Verification items for the finished model (mm, model axes). Face numbers are marked on the shaded views. A direction names the side the tool comes from. Round coordinates to 2 decimals unless told otherwise and drop trailing zeros. Write each loop counter-clockwise with the first axis right and the second up, starting at its lowest first coordinate (ties: lowest second). Pieces come first, ordered by that corner, then holes. Notation, with made-up numbers: (60, 3) - (110, 3) arc R21 ccw to (110, 8) - close; hole circle Ø3 at (-39.5, -38.5). An arc over 180 degrees is marked (long way). Answer as a JSON object with one key per item and string values.
```python
from build123d import *

# Parameters (mm, degrees)
BOSS_EXTRUDE1_DEPTH = 35.56
SKETCH3_W           = 35.56
SKETCH3_H           = 6.35
BOSS_EXTRUDE2_DEPTH = 50.8
BOSS_EXTRUDE4_DEPTH = 35.56
CUT_EXTRUDE1_DEPTH  = 45.72
FILLET5_R           = 2.54


with BuildPart() as part:
    # Sketch2 → Boss-Extrude1 (new body)
    with BuildSketch(Plane.XY):
        Polygon((0, 0), (-114.3, 0), (-33.47769491, 80.82230509), (-28.98756685, 76.332177029), (-98.969743879, 6.35), (0, 6.35), align=None)
    extrude(amount=BOSS_EXTRUDE1_DEPTH)

    # Sketch3 → Boss-Extrude2 (add)
    with BuildSketch(Plane(origin=(-57.15, 57.15, 0), x_dir=(0, 0, 1), z_dir=(-0.707106781186544, 0.7071067811865511, 0))):
        with Locations((17.78, -42.08730509)):
            Rectangle(SKETCH3_W, SKETCH3_H)
    extrude(amount=BOSS_EXTRUDE2_DEPTH)

    # Sketch5 → Boss-Extrude4 (add)
    with BuildSketch(Plane.XY.offset(35.56)):
        Polygon((-98.969743879, 6.35), (-63.978655364, 41.341088515), (-63.978655364, 6.35), align=None)
    extrude(amount=-BOSS_EXTRUDE4_DEPTH)

    # Sketch6 → Cut-Extrude1 (cut)
    with BuildSketch(Plane(origin=(0, 0, 0), x_dir=(-1, 0, 0), z_dir=(0, 0, -1))):
        Polygon((67.153655364, 42.656216575), (67.153655364, 9.525), (100.284871939, 9.525), align=None)
    extrude(amount=-CUT_EXTRUDE1_DEPTH, mode=Mode.SUBTRACT)

    # Fillet5
    fillet5_edges = [part.edges().sort_by_distance(p)[0] for p in [
        (0, 0, 17.78),
        (-114.3, 0, 17.78),
        (-33.47769491, 80.82230509, 17.78),
        (-28.98756685, 76.332177029, 17.78),
        (0, 6.35, 17.78),
        (-31.23263088, 78.577241059, 35.56),
        (-101.727641431, 12.572358569, 0),
        (-101.727641431, 12.572358569, 35.56),
        (-59.071424855, 55.228575145, 35.56),
        (-102.625667043, 47.595357442, 0),
        (-89.155282861, 25.144717139, 17.78),
        (-107.115795103, 43.105229381, 0),
        (-107.115795103, 43.105229381, 35.56),
        (-84.6651548, 29.6348452, 17.78),
        (-102.625667043, 47.595357442, 35.56),
        (-122.831243315, 63.310805654, 0),
        (-125.076307345, 61.065741623, 17.78),
        (-122.831243315, 63.310805654, 35.56),
        (-120.586179285, 65.555869684, 17.78),
        (-57.15, 0, 35.56),
        (-46.483111107, 58.836632772, 0),
        (-46.483111107, 58.836632772, 35.56),
        (-63.978655364, 6.35, 17.78),
        (-63.978655364, 23.845544257, 0),
        (-63.978655364, 41.341088515, 17.78),
        (-63.978655364, 23.845544257, 35.56),
        (-67.153655364, 42.656216575, 17.78),
        (-100.284871939, 9.525, 17.78),
        (-67.153655364, 9.525, 17.78),
        (0, 3.175, 35.56),
        (-57.15, 0, 0),
        (-59.071424855, 55.228575145, 0),
        (-31.23263088, 78.577241059, 0),
        (-31.989327682, 6.35, 0),
        (0, 3.175, 0),
        (-31.989327682, 6.35, 35.56),
    ]]
    fillet(fillet5_edges, radius=FILLET5_R)


solid = part.part
```
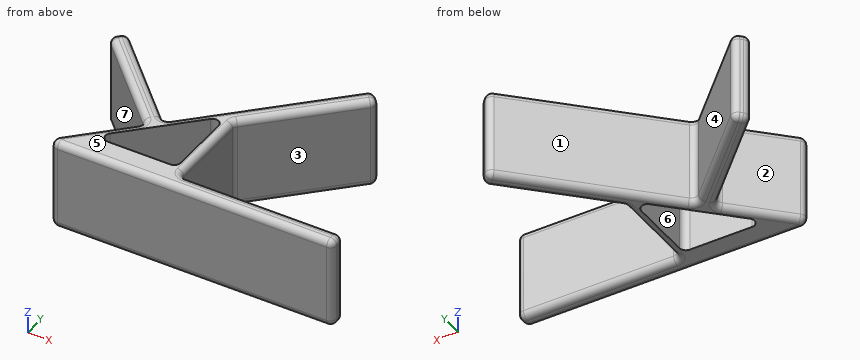
1. Mould release check, pull along Y, two halves, no side actions. Record for the marked faces 4, 5, 6 and 7: released by +Y, released by -Y, zero draft, split by the parting line, or undercut.
Completed:
{"face 4": "released by +Y", "face 5": "zero draft", "face 6": "undercut", "face 7": "undercut"}
2. Cross-section at B-B (x = -23.5). Record the boundary of the cut face in (y, z), plus the area to 3 significant figures.
Completed:
{"outline": "(0, 2.54) arc R2.54 ccw to (2.54, 0) - (3.81, 0) arc R2.54 ccw to (6.35, 2.54) - (6.35, 33.02) arc R2.54 ccw to (3.81, 35.56) - (2.54, 35.56) arc R2.54 ccw to (0, 33.02) - close", "area": "220 mm^2"}
3. Cross-section at A-A (z = 25). Record the boundary of the cut face in (x, y) (3 decimals), plus the area to 3 significant figures.
Completed:
{"outline": "(-123.28, 59.27) - (-90.951, 26.941) arc R2.54 cw to (-90.951, 23.349) - (-109.964, 4.336) arc R2.54 ccw to (-108.168, 0) - (-2.54, 0) arc R2.54 ccw to (0, 2.54) - (0, 3.81) arc R2.54 ccw to (-2.54, 6.35) - (-61.439, 6.35) arc R2.54 cw to (-63.979, 8.89) - (-63.979, 40.289) arc R2.54 cw to (-63.235, 42.085) - (-30.784, 74.536) arc R2.54 ccw to (-30.784, 78.128) - (-31.682, 79.026) arc R2.54 ccw to (-35.274, 79.026) - (-82.869, 31.431) arc R2.54 cw to (-86.461, 31.431) - (-118.79, 63.76) arc R2.54 ccw to (-122.382, 63.76) - (-123.28, 62.862) arc R2.54 ccw to start; hole (-95.949, 13.861) arc R2.54 ccw to (-94.153, 9.525) - (-69.694, 9.525) arc R2.54 ccw to (-67.154, 12.065) - (-67.154, 36.524) arc R2.54 ccw to (-71.49, 38.32) - close", "area": "1,750 mm^2"}
4. Go/stop test with flat-tipped pins: pin 1 (4 mm diameter, centred on x = -76.5, z = 31.5, fed in from +Y); pin 2 (12 mm diameter, centred on y = 27, z = 24.5, fed in from -X); pin 3 (6 mm diameter, centred on y = 15, z = 22, fed in from -X); pin 4 (12 mm diameter, centred on x = -13, y = 15.5, fed in from -Z). Record where each tip stops, or that it passes through.
Completed:
{"pin 1": "stops at y = 39.8", "pin 2": "stops at x = -97.01", "pin 3": "stops at x = -102.3", "pin 4": "passes through"}
5. Access from +Z, -Z, +X, -X, +Y, -Y to the whole of each face (thin tool, end or side, straight path). Record for the marked faces 1, 2 and 3.
Completed:
{"face 1": "+Z, -Z, +Y", "face 2": "+Z, -Z, -X", "face 3": "+Z, -Z, +X"}
6. Material ranges on probe 1 along Y at (x, z) = (-91.5, 22) (3 decimals); probe 2 along Y at (x, z) = (-80, 32) (3 decimals); probe 3 along Y at (x, z) = (-9, 7.5), recorded low to high. Write a range as from..to.
Completed:
{"probe 1": "y = 0..9.525, 18.31..22.8, 27.489..36.47", "probe 2": "y = 0..9.525, 29.81..34.3", "probe 3": "y = 0..6.35"}
